Input: dimensioned drawing with shaded views. Units: mm. Origin: part minimum x, y, z. A direction names the side the tool comes from. Coordinates: 2 decimals unless noted, no trailing zeros. Order: outer loops, then holes, each group sorted by start corner. A loop starts at its lowest first (then second) coordinate and runs counter-clockwise, first axis right, second up. Notation, with made-up numbers: (-35, -7) -> (-12, -7) arc R18 ccw to (-12, 12) -> close; hole circle Ø9 at (71.25, 28). An arc over 180 degrees is marked (long way). Answer in a Markdown table with one row per item. Add a question column.
1) Contact query for flat-ended pins moving along their axis: P1, Ø3, axis at x = 41.5, y = 6, coming from the -Z side; P2, Ø5, axis at y = 4, z = 22.5, coming from the -X side; P3, Ø1.5, axis at x = 64.5, z = 54.5, coming from the -Y side. Output: stop coordinate, or through.
2) Section query C-C on z = 60.5. Return the cut outline in (x, y), then the cut area to 3 significant figures.
3) Section query A-A on y = 5. Return the cut outline in (x, z), then the cut area to 3 significant figures.
4) Ray query, line 1 (X direction, y = 1.5, z = 55); line 2 (Z direction, x = 85.5, y = 2); line 3 (Z direction, x = 55, y = 1.25). Return the intervals inside material, ascending. Write a range as from..to.
5) Set-up query: the marked faces 1 and 2. Return all of +Z, -Z, +X, -X, +Y, -Y with unobstructed straight access to the full face (end or side cutting, diameter ignored); none if empty.
6) Section query B-B on x = 66.5. Return the cut outline in (y, z).
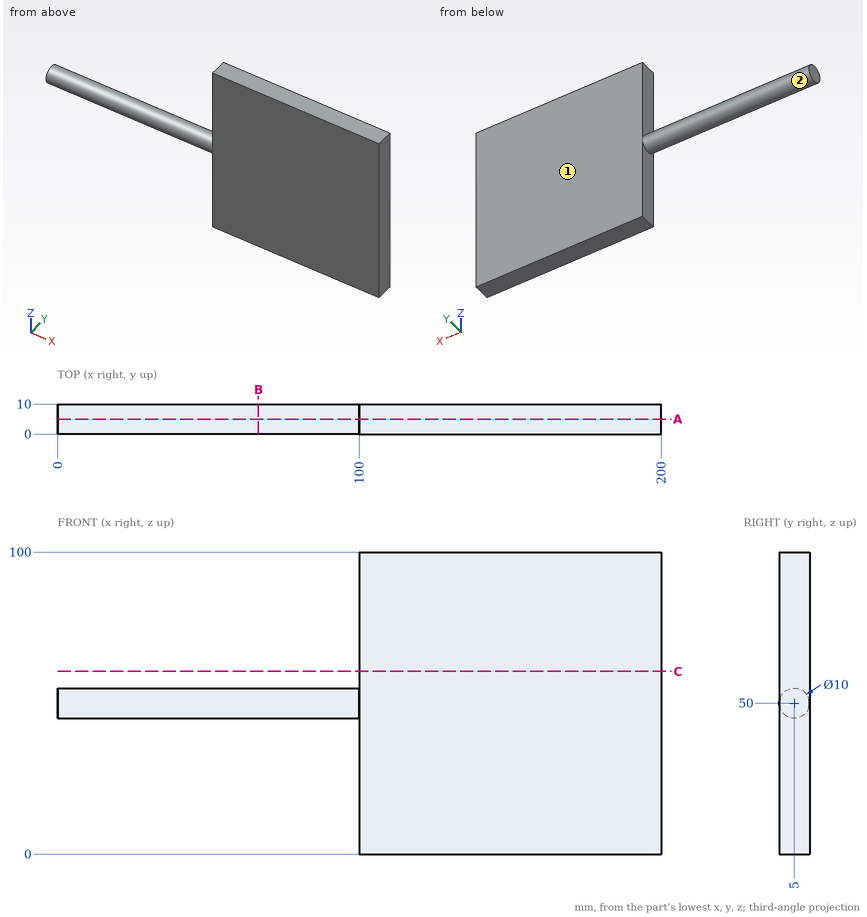
Result:
| question | item | result |
|---|---|---|
| 1 | P1 | z = 45 |
| 1 | P2 | x = 100 |
| 1 | P3 | y = 1.69 |
| 2 | outline | (100, 0) -> (200, 0) -> (200, 10) -> (100, 10) -> close |
| 2 | area | 1,000 mm2 |
| 3 | outline | (0, 45) -> (100, 45) -> (100, 0) -> (200, 0) -> (200, 100) -> (100, 100) -> (100, 55) -> (0, 55) -> close |
| 3 | area | 11,000 mm2 |
| 4 | line 1 | 100..200 |
| 4 | line 2 | 46..54 |
| 4 | line 3 | 46.69..53.31 |
| 5 | face 1 | +Z, -Z, +X, -X, +Y |
| 5 | face 2 | -X |
| 6 | outline | circle Ø10 at (5, 50) |
